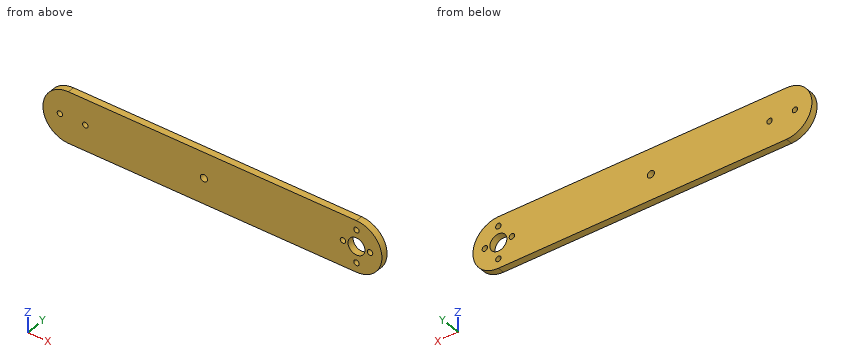
```python
from build123d import *

# Parameters (mm, degrees)
SKETCH2_R           = 5
SKETCH2_R_2         = 1.6
BOSS_EXTRUDE1_DEPTH = 4
SKETCH3_R           = 2.1
CUT_EXTRUDE1_DEPTH  = 186.650208726


with BuildPart() as part:
    # Sketch2 → Boss-Extrude1 (new body)
    with BuildSketch(Plane(origin=(0, 0, 0), x_dir=(1, 0, 0), z_dir=(0, 1, 0))):
        with BuildLine():
            Line((0, -15), (-170, -15))
            ThreePointArc((-170, -15), (-185, 0), (-170, 15))
            Line((-170, 15), (0, 15))
            ThreePointArc((0, 15), (15, 0), (0, -15))
        make_face()
        with Locations(Location((0, 0, 0), (0, 0, 270))):
            Circle(SKETCH2_R, mode=Mode.SUBTRACT)
        with Locations(Location((8, 0, 0), (0, 0, 270))):
            Circle(SKETCH2_R_2, mode=Mode.SUBTRACT)
        with Locations(Location((-160, 0, 0), (0, 0, 270))):
            Circle(SKETCH2_R_2, mode=Mode.SUBTRACT)
        with Locations(Location((-175, 0, 0), (0, 0, 270))):
            Circle(SKETCH2_R_2, mode=Mode.SUBTRACT)
        with Locations(Location((0, -9.5, 0), (0, 0, 270))):
            Circle(SKETCH2_R_2, mode=Mode.SUBTRACT)
        with Locations(Location((0, 9.5, 0), (0, 0, 270))):
            Circle(SKETCH2_R_2, mode=Mode.SUBTRACT)
        with Locations(Location((-8, 0, 0), (0, 0, 270))):
            Circle(SKETCH2_R_2, mode=Mode.SUBTRACT)
    extrude(amount=BOSS_EXTRUDE1_DEPTH)

    # Sketch3 → Cut-Extrude1 (cut, through all)
    with BuildSketch(Plane(origin=(0, 4, 0), x_dir=(1, 0, 0), z_dir=(0, 1, 0))):
        with Locations(Location((-90, 0, 0), (0, 0, 270))):
            Circle(SKETCH3_R)
    extrude(amount=-CUT_EXTRUDE1_DEPTH, mode=Mode.SUBTRACT)


solid = part.part
```
Part model, mm, in its own coordinate system. Round coordinates to 2 decimals unless told otherwise and drop trailing zeros. Loops run counter-clockwise (first coordinate to the right, second up) from the corner with the lowest first, then second, coordinate; pieces in that order, holes last. Notation, with made-up numbers: (4.5, 45) -> (10.5, 45) arc R32 cw to (10.5, 80) -> close; hole circle Ø10 at (40.25, 25). An arc over 180 degrees is marked (long way). Use CSV: the item, a comma, the result in double quotes. Start each with the question number.
1) Cut at B-B, the plane y = 1.8. Give the number of separate pieces and of enclosed holes in the cut face, plus the area to 3 significant figures.
2) Wall check: L1, parallel to X at y = 0.4, z = 3.5; L2, parallel to X at y = 2.05, z = -9.5; L3, parallel to X at y = 1.9, z = -6.5. Give the ranges that are in metal, low to high. Write a range as [from, to].
3) Cut at A-A, the plane x = -90. Write the cut outline in (y, z), plus the area to 3 significant figures.
Determined:
1,separate pieces,"1"
1,enclosed holes,"8"
1,area,"5,670 mm2"
2,L1,"x = [-184.59, -3.57], [3.57, 14.59]"
2,L2,"x = [-181.61, -1.6], [1.6, 11.61]"
2,L3,"x = [-183.52, 13.52]"
3,outline,"(0, -15) -> (4, -15) -> (4, -2.1) -> (0, -2.1) -> close; (0, 2.1) -> (4, 2.1) -> (4, 15) -> (0, 15) -> close"
3,area,"103 mm2"
